Could you check a few things on this model? Use its own coordinates, in mm. A direction names the side the tool comes from. Round coordinates to 2 decimals unless told otherwise and drop trailing zeros. Write each loop counter-clockwise with the first axis right and the second up, starting at its lowest first coordinate (ties: lowest second). Pieces come first, ordered by that corner, then holes. Notation, with made-up numbers: (74, -30) -> (91, -30) arc R8 ccw to (91, -18) -> close; hole circle Ø1 at (16.25, 20.5). An arc over 180 degrees is marked (long way). Answer in a Markdown table with one row per item.
from build123d import *

# Parameters (mm, degrees)
SKETCH1_W           = 100
SKETCH1_H           = 110
BOSS_EXTRUDE1_DEPTH = 70
SKETCH2_W           = 60
SKETCH2_H           = 10
CUT_EXTRUDE1_DEPTH  = 70
CUT_EXTRUDE2_DEPTH  = 70
SKETCH4_R           = 10
CUT_EXTRUDE3_DEPTH  = 30
SKETCH5_W           = 100
SKETCH5_H           = 10
CUT_EXTRUDE4_DEPTH  = 185
SKETCH7_W           = 60
SKETCH7_H           = 10
CUT_EXTRUDE5_DEPTH  = 200
SKETCH8_R           = 25
SKETCH8_R_2         = 10
BOSS_EXTRUDE3_DEPTH = 20
SKETCH9_R           = 25
CUT_EXTRUDE7_DEPTH  = 40
CUT_EXTRUDE8_DEPTH  = 30
SKETCH11_W          = 60
SKETCH11_H          = 10
CUT_EXTRUDE9_DEPTH  = 130
SKETCH12_W          = 30
SKETCH12_H          = 10
CUT_EXTRUDE10_DEPTH = 130


with BuildPart() as part:
    # Sketch1 → Boss-Extrude1 (new body)
    with BuildSketch(Plane.XY):
        with Locations((50, 55)):
            Rectangle(SKETCH1_W, SKETCH1_H)
    extrude(amount=BOSS_EXTRUDE1_DEPTH)

    # Sketch2 → Cut-Extrude1 (cut)
    with BuildSketch(Plane.XY.offset(70)):
        with Locations((50, 5)):
            Rectangle(SKETCH2_W, SKETCH2_H)
    extrude(amount=-CUT_EXTRUDE1_DEPTH, mode=Mode.SUBTRACT)

    # Sketch3 → Cut-Extrude2 (cut)
    with BuildSketch(Plane.XY.offset(70)):
        with BuildLine():
            Line((0, 110), (0, 60))
            ThreePointArc((0, 60), (14.644660941, 95.355339059), (50, 110))
            Line((50, 110), (0, 110))
        make_face()
        with BuildLine():
            Line((100, 110), (50, 110))
            ThreePointArc((50, 110), (85.355339059, 95.355339059), (100, 60))
            Line((100, 60), (100, 110))
        make_face()
    extrude(amount=-CUT_EXTRUDE2_DEPTH, mode=Mode.SUBTRACT)

    # Sketch4 → Cut-Extrude3 (cut)
    with BuildSketch(Plane(origin=(0, 0, 0), x_dir=(-1, 0, 0), z_dir=(0, 0, -1))):
        with Locations((-50, 60)):
            Circle(SKETCH4_R)
    extrude(amount=-CUT_EXTRUDE3_DEPTH, mode=Mode.SUBTRACT)

    # Sketch5 → Cut-Extrude4 (cut)
    with BuildSketch(Plane.XZ):
        with Locations((50, 5)):
            Rectangle(SKETCH5_W, SKETCH5_H)
    extrude(amount=-CUT_EXTRUDE4_DEPTH, mode=Mode.SUBTRACT)

    # Sketch7 → Cut-Extrude5 (cut)
    with BuildSketch(Plane(origin=(0, 10, 0), x_dir=(-1, 0, 0), z_dir=(0, -1, 0))):
        with Locations((-50, -15)):
            Rectangle(SKETCH7_W, SKETCH7_H)
    extrude(amount=-CUT_EXTRUDE5_DEPTH, mode=Mode.SUBTRACT)

    # Sketch8 → Boss-Extrude3 (add)
    with BuildSketch(Plane(origin=(0, 0, 20), x_dir=(-1, 0, 0), z_dir=(0, 0, -1))):
        with Locations((-50, 60)):
            Circle(SKETCH8_R)
        with Locations((-50, 60)):
            Circle(SKETCH8_R_2, mode=Mode.SUBTRACT)
    extrude(amount=BOSS_EXTRUDE3_DEPTH)

    # Sketch9 → Cut-Extrude7 (cut)
    with BuildSketch(Plane.XY.offset(70)):
        with Locations((50, 60)):
            Circle(SKETCH9_R)
    extrude(amount=-CUT_EXTRUDE7_DEPTH, mode=Mode.SUBTRACT)

    # Sketch10 → Cut-Extrude8 (cut)
    with BuildSketch(Plane.XY.offset(70)):
        with BuildLine():
            Line((25, 103.301270189), (25, 60))
            ThreePointArc((25, 60), (50, 85), (75, 60))
            Line((75, 60), (75, 103.301270189))
            ThreePointArc((75, 103.301270189), (50, 110), (25, 103.301270189))
        make_face()
    extrude(amount=-CUT_EXTRUDE8_DEPTH, mode=Mode.SUBTRACT)

    # Sketch11 → Cut-Extrude9 (cut)
    with BuildSketch(Plane(origin=(0, 10, 0), x_dir=(-1, 0, 0), z_dir=(0, -1, 0))):
        with Locations((-50, -65)):
            Rectangle(SKETCH11_W, SKETCH11_H)
    extrude(amount=-CUT_EXTRUDE9_DEPTH, mode=Mode.SUBTRACT)

    # Sketch12 → Cut-Extrude10 (cut)
    with BuildSketch(Plane.XZ.offset(-10)):
        with Locations((50, 55)):
            Rectangle(SKETCH12_W, SKETCH12_H)
    extrude(amount=-CUT_EXTRUDE10_DEPTH, mode=Mode.SUBTRACT)


solid = part.part
1) Imagine slicing it at A-A, the plane z = 16. Please give me the cut outline in (x, y), plus the area to 3 significant figures.
Findings:
| item | result |
|---|---|
| outline | (0, 0) -> (20, 0) -> (20, 100) arc R50 ccw to (0, 60) -> close; circle Ø50 at (50, 60); (80, 0) -> (100, 0) -> (100, 60) arc R50 ccw to (80, 100) -> close; hole circle Ø20 at (50, 60) |
| area | 5,170 mm^2 |
2) Thinking about a two-plate mould opening in X: for faces 1 (the face through (80, 38.2, 60.4)), 2 (the face through (90, 0, 40)), 3 (the face through (100, 30, 40)), which applies, +X half, -X half, draft (parallel to the pull), parting line (faces both ways), or undercut?
Findings:
| item | result |
|---|---|
| face 1 | undercut |
| face 2 | draft |
| face 3 | +X half |
3) Imagine slicing it at D-D, the plane z = 38.5. Please give me the cut outline in (x, y).
Findings:
| item | result |
|---|---|
| outline | (0, 0) -> (20, 0) -> (20, 10) -> (80, 10) -> (80, 0) -> (100, 0) -> (100, 60) arc R50 ccw to (0, 60) -> close; hole circle Ø50 at (50, 60) |
4) Imagine slicing it at C-C, the plane y = 82. Please give me the cut outline in (x, z), plus the area to 3 significant figures.
Findings:
| item | result |
|---|---|
| outline | (5.1, 10) -> (20, 10) -> (20, 20) -> (38.13, 20) -> (38.13, 0) -> (61.87, 0) -> (61.87, 20) -> (80, 20) -> (80, 10) -> (94.9, 10) -> (94.9, 70) -> (80, 70) -> (80, 60) -> (75, 60) -> (75, 40) -> (61.87, 40) -> (61.87, 30) -> (38.13, 30) -> (38.13, 40) -> (25, 40) -> (25, 60) -> (20, 60) -> (20, 70) -> (5.1, 70) -> close |
| area | 3,430 mm^2 |
5) Imagine slicing it at B-B, the plane z = 53. Please give me the cut outline in (x, y), plus the area to 3 significant figures.
Findings:
| item | result |
|---|---|
| outline | (0, 0) -> (20, 0) -> (20, 10) -> (35, 10) -> (35, 40) arc R25 cw to (25, 60) -> (25, 103.3) arc R50 ccw to (0, 60) -> close; (65, 10) -> (80, 10) -> (80, 0) -> (100, 0) -> (100, 60) arc R50 ccw to (75, 103.3) -> (75, 60) arc R25 cw to (65, 40) -> close |
| area | 5,160 mm^2 |
6) Please list where these lines run through material, in increasing order: line 1 (X direction, y = 29, z = 67); line 2 (Y direction, x = 50, z = 14); line 3 (Y direction, x = 50, z = 37).
Findings:
| item | result |
|---|---|
| line 1 | x = 0 to 20, 80 to 100 |
| line 2 | y = 35 to 50, 70 to 85 |
| line 3 | y = 10 to 35, 85 to 110 |
7) For pin 1 (25 mm diameter, centred on x = 38, y = 48.5, fed in from +Z); pin 2 (6 mm diameter, centred on y = 85, z = 50, fed in from -X); pin 3 (20 mm diameter, centred on x = 39.5, z = 46, fed in from -Y), each with a flat end and sliding along its axis, tell me the tip position at first contact or that it passes through.
Findings:
| item | result |
|---|---|
| pin 1 | stops at z = 60 |
| pin 2 | stops at x = 5.1 |
| pin 3 | stops at y = 10 |
8) For faces 4 (the face through (74, 46, 60)), 5 (the face through (44.58, 35.594, 41.877)), 6 (the face through (20, 38.2, 60.4)), which set-ups out of +Z, -Z, +X, -X, +Y, -Y let a thin tool reach every point of the face, with its end or its side?
Findings:
| item | result |
|---|---|
| face 4 | +Z, +Y, -Y |
| face 5 | +Z |
| face 6 | -Y |
